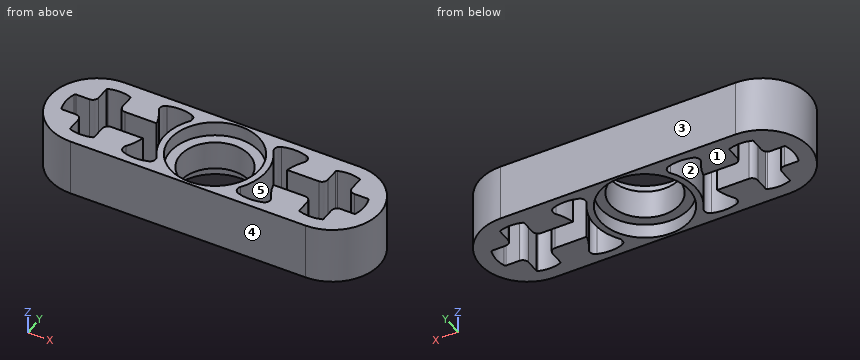
```python
from build123d import *

# Parameters (mm, degrees)
SKETCH2_R           = 2.4
BOSS_EXTRUDE1_DEPTH = 2
SKETCH4_R           = 3.1
CUT_EXTRUDE1_DEPTH  = 1


with BuildPart() as part:
    # Sketch2 → Boss-Extrude1 (new, symmetric)
    with BuildSketch(Plane.XY):
        with BuildLine():
            Line((8.2, 3.3), (-8.2, 3.3))
            ThreePointArc((-8.2, 3.3), (-11.5, 0), (-8.2, -3.3))
            Line((-8.2, -3.3), (8.2, -3.3))
            ThreePointArc((8.2, -3.3), (11.5, 0), (8.2, 3.3))
        make_face()
        with BuildLine():
            Line((-10.177705214, 0.84), (-9.24, 0.84))
            ThreePointArc((-9.24, 0.84), (-8.957157288, 0.957157288), (-8.84, 1.24))
            Line((-8.84, 1.24), (-8.84, 2.177705214))
            ThreePointArc((-8.84, 2.177705214), (-8.821293884, 2.235940121), (-8.772173913, 2.27238805))
            ThreePointArc((-8.772173913, 2.27238805), (-8, 2.4), (-7.227826087, 2.27238805))
            ThreePointArc((-7.227826087, 2.27238805), (-7.178706116, 2.235940121), (-7.16, 2.177705214))
            Line((-7.16, 2.177705214), (-7.16, 1.24))
            ThreePointArc((-7.16, 1.24), (-7.042842712, 0.957157288), (-6.76, 0.84))
            Line((-6.76, 0.84), (-5.822294786, 0.84))
            Line((-5.822294786, 0.84), (-5.751800721, 0.84))
            Line((-5.751800721, 0.84), (-4.55081169, 0.84))
            ThreePointArc((-4.55081169, 0.84), (-4.757752494, 1.445797742), (-5.070126582, 2.004580194))
            ThreePointArc((-5.070126582, 2.004580194), (-5.119033599, 2.358251088), (-4.865957447, 2.610099174))
            ThreePointArc((-4.865957447, 2.610099174), (-4, 2.75), (-3.134042553, 2.610099174))
            ThreePointArc((-3.134042553, 2.610099174), (-2.880966401, 2.358251088), (-2.929873418, 2.004580194))
            ThreePointArc((-2.929873418, 2.004580194), (-3.55, 0), (-2.929873418, -2.004580194))
            ThreePointArc((-2.929873418, -2.004580194), (-2.880966401, -2.358251088), (-3.134042553, -2.610099174))
            ThreePointArc((-3.134042553, -2.610099174), (-4, -2.75), (-4.865957447, -2.610099174))
            ThreePointArc((-4.865957447, -2.610099174), (-5.119033599, -2.358251088), (-5.070126582, -2.004580194))
            ThreePointArc((-5.070126582, -2.004580194), (-4.757752494, -1.445797742), (-4.55081169, -0.84))
            Line((-4.55081169, -0.84), (-5.751800721, -0.84))
            Line((-5.751800721, -0.84), (-5.822294786, -0.84))
            Line((-5.822294786, -0.84), (-6.76, -0.84))
            ThreePointArc((-6.76, -0.84), (-7.042842712, -0.957157288), (-7.16, -1.24))
            Line((-7.16, -1.24), (-7.16, -2.177705214))
            ThreePointArc((-7.16, -2.177705214), (-7.178706116, -2.235940121), (-7.227826087, -2.27238805))
            ThreePointArc((-7.227826087, -2.27238805), (-8, -2.4), (-8.772173913, -2.27238805))
            ThreePointArc((-8.772173913, -2.27238805), (-8.821293884, -2.235940121), (-8.84, -2.177705214))
            Line((-8.84, -2.177705214), (-8.84, -1.24))
            ThreePointArc((-8.84, -1.24), (-8.957157288, -0.957157288), (-9.24, -0.84))
            Line((-9.24, -0.84), (-10.177705214, -0.84))
            ThreePointArc((-10.177705214, -0.84), (-10.235940121, -0.821293884), (-10.27238805, -0.772173913))
            ThreePointArc((-10.27238805, -0.772173913), (-10.4, 0), (-10.27238805, 0.772173913))
            ThreePointArc((-10.27238805, 0.772173913), (-10.235940121, 0.821293884), (-10.177705214, 0.84))
        make_face(mode=Mode.SUBTRACT)
        Circle(SKETCH2_R, mode=Mode.SUBTRACT)
        with BuildLine():
            Line((8.84, 2.177705214), (8.84, 1.24))
            ThreePointArc((8.84, 1.24), (8.957157288, 0.957157288), (9.24, 0.84))
            Line((9.24, 0.84), (10.177705214, 0.84))
            ThreePointArc((10.177705214, 0.84), (10.235940121, 0.821293884), (10.27238805, 0.772173913))
            ThreePointArc((10.27238805, 0.772173913), (10.4, 0), (10.27238805, -0.772173913))
            ThreePointArc((10.27238805, -0.772173913), (10.235940121, -0.821293884), (10.177705214, -0.84))
            Line((10.177705214, -0.84), (9.24, -0.84))
            ThreePointArc((9.24, -0.84), (8.957157288, -0.957157288), (8.84, -1.24))
            Line((8.84, -1.24), (8.84, -2.177705214))
            ThreePointArc((8.84, -2.177705214), (8.821293884, -2.235940121), (8.772173913, -2.27238805))
            ThreePointArc((8.772173913, -2.27238805), (8, -2.4), (7.227826087, -2.27238805))
            ThreePointArc((7.227826087, -2.27238805), (7.178706116, -2.235940121), (7.16, -2.177705214))
            Line((7.16, -2.177705214), (7.16, -1.24))
            ThreePointArc((7.16, -1.24), (7.042842712, -0.957157288), (6.76, -0.84))
            Line((6.76, -0.84), (5.822294786, -0.84))
            Line((5.822294786, -0.84), (5.751800721, -0.84))
            Line((5.751800721, -0.84), (4.55081169, -0.84))
            ThreePointArc((4.55081169, -0.84), (4.757752494, -1.445797742), (5.070126582, -2.004580194))
            ThreePointArc((5.070126582, -2.004580194), (5.119033599, -2.358251088), (4.865957447, -2.610099174))
            ThreePointArc((4.865957447, -2.610099174), (4, -2.75), (3.134042553, -2.610099174))
            ThreePointArc((3.134042553, -2.610099174), (2.880966401, -2.358251088), (2.929873418, -2.004580194))
            ThreePointArc((2.929873418, -2.004580194), (3.55, 0), (2.929873418, 2.004580194))
            ThreePointArc((2.929873418, 2.004580194), (2.880966401, 2.358251088), (3.134042553, 2.610099174))
            ThreePointArc((3.134042553, 2.610099174), (4, 2.75), (4.865957447, 2.610099174))
            ThreePointArc((4.865957447, 2.610099174), (5.119033599, 2.358251088), (5.070126582, 2.004580194))
            ThreePointArc((5.070126582, 2.004580194), (4.757752494, 1.445797742), (4.55081169, 0.84))
            Line((4.55081169, 0.84), (5.751800721, 0.84))
            Line((5.751800721, 0.84), (5.822294786, 0.84))
            Line((5.822294786, 0.84), (6.76, 0.84))
            ThreePointArc((6.76, 0.84), (7.042842712, 0.957157288), (7.16, 1.24))
            Line((7.16, 1.24), (7.16, 2.177705214))
            ThreePointArc((7.16, 2.177705214), (7.178706116, 2.235940121), (7.227826087, 2.27238805))
            ThreePointArc((7.227826087, 2.27238805), (8, 2.4), (8.772173913, 2.27238805))
            ThreePointArc((8.772173913, 2.27238805), (8.821293884, 2.235940121), (8.84, 2.177705214))
        make_face(mode=Mode.SUBTRACT)
    extrude(amount=BOSS_EXTRUDE1_DEPTH, both=True)

    # Sketch4 → Cut-Extrude1 (cut)
    with BuildSketch(Plane.XY.offset(2)):
        Circle(SKETCH4_R)
    cut_extrude1 = extrude(amount=-CUT_EXTRUDE1_DEPTH, mode=Mode.SUBTRACT)

    # Mirror1: Cut-Extrude1 across plane
    add(cut_extrude1.mirror(Plane.XY), mode=Mode.SUBTRACT)


solid = part.part
```
Geometry check sheet. Reference: the model listing, model coordinates, mm. Face numbers are marked on the shaded views. A direction names the side the tool comes from. Give positions to 0.01 mm unless a question says otherwise; leave off trailing zeros. Order: outer loops, then holes, each group sorted by start corner. A loop starts at its lowest first (then second) coordinate and runs counter-clockwise, first axis right, second up.
1. Section check B-B, the plane x = 6.5. Enter the section's corners in (y, z).
2. Gauge pin test, flat ends, axial feed: pin 1 Ø0.5 at (y, z) = (-1.5, 0) entering from +X; pin 2 Ø0.5 at (x, z) = (9.5, -0.5) entering from -Y; pin 3 Ø0.5 at (y, z) = (1.5, -1) entering from -X; pin 4 Ø3 at (x, y) = (0.5, 0) entering from -Z. Record the tip position at first contact, or that the pin passes through.
3. Section check C-C, the plane y = 1.5. Give the number of separate pieces and of enclosed holes in the cut face, and give its area (3 significant figures).
4. Thickness scan on L1, parallel to Y at x = 0, z = 0.45; L2, parallel to X at y = -1, z = 1.3; L3, parallel to Y at x = 0, z = -1.4. Record the ranges inside material, lowest first.
5. Access from +Z, -Z, +X, -X, +Y, -Y to the whole of each face (thin tool, end or side, straight path). Record for the marked faces 4 and 5.
6. Release check for a two-part mould opening along Y. For the marked faces 1, 2 and 3 record: pulls with the +Y half, pulls with the -Y half, needs draft (parallel to the pull), parting line crosses it, or undercut.
7. Section check A-A, the plane y = 0. Enter the section's corners in (x, z), and give its area (3 significant figures).
Values follow:
1. outline: (-3.3, -2) - (-0.84, -2) - (-0.84, 2) - (-3.3, 2) - close; (0.84, -2) - (3.3, -2) - (3.3, 2) - (0.84, 2) - close
2. pin 1: stops at x = 11.25
2. pin 2: stops at y = -3.13
2. pin 3: stops at x = -11.25
2. pin 4: passes through
3. separate pieces: 6
3. enclosed holes: 0
3. area: 44.8 mm2
4. L1: y = -3.3 to -2.4, 2.4 to 3.3
4. L2: x = -11.34 to -8.92, -7.08 to -4.59, -3.41 to -2.93, 2.93 to 3.41, 4.59 to 7.08, 8.92 to 11.34
4. L3: y = -3.3 to -3.1, 3.1 to 3.3
5. face 4: +Z, -Z, +X, -X, -Y
5. face 5: +Z, -Z
6. face 1: needs draft
6. face 2: undercut
6. face 3: pulls with the +Y half
7. outline: (-11.5, -2) - (-10.4, -2) - (-10.4, 2) - (-11.5, 2) - close; (-3.55, -2) - (-3.1, -2) - (-3.1, -1) - (-2.4, -1) - (-2.4, 1) - (-3.1, 1) - (-3.1, 2) - (-3.55, 2) - close; (2.4, -1) - (3.1, -1) - (3.1, -2) - (3.55, -2) - (3.55, 2) - (3.1, 2) - (3.1, 1) - (2.4, 1) - close; (10.4, -2) - (11.5, -2) - (11.5, 2) - (10.4, 2) - close
7. area: 15.2 mm2
